Geometry check sheet. Reference: the model listing, model coordinates, mm. A direction names the side the tool comes from. Give positions to 0.01 mm unless a question says otherwise; leave off trailing zeros. Write each loop counter-clockwise with the first axis right and the second up, starting at its lowest first coordinate (ties: lowest second). Pieces come first, ordered by that corner, then holes.
(1) Mould release check, pull along X, two halves, no side actions. Record for faces 3 (the cylindrical face through (-1.923, 3.131, 107.933)), 4 (the flat face through (50.8, 3, -67)), 5 (the flat face through (-1, 6.35, -2)): +X half, -X half, draft (parallel to the pull), parting line (faces both ways), or undercut.
(2) Cross-section at A-A (x = 0). Record the boundary of the cut face in (y, z).
(3) Thickness scan on line 1 along Z through (x, y) = (-65.5, 3.5); line 2 along Z through (x, y) = (-7.5, 1); line 3 along X through (y, z) = (4.5, -36.83) (3 decimals). Record the ranges inside material, lowest first.
(4) Cross-section at D-D (y = 3). Count the separate pieces of the cut face and the enclosed holes in it, and give its area (3 significant figures).
(5) Depth check by flat-ended pin: P1, Ø1.5, axis at x = -40.5, y = 4.5, coming from the -Z side; P2, Ø3, axis at x = -45, y = 4, coming from the -Z side; P3, Ø3, axis at y = 4.5, z = -67, coming from the +X side. Enter the tip coordinate at first touch or a pass-through.
(6) Tool access check on faces 1 (the flat face through (-41, 3, -12.7)), 2 (the cylindrical face through (82.554, 3.131, 0.435)). Record the directions out of +Z, -Z, +X, -X, +Y, -Y that give a thin tool (end or side, any length) a straight path to the whole face; none if there is none.
(7) Cross-section at C-C (z = -21). Record the boundary of the cut face in (x, y), and give its area (3 significant figures).
(8) Cross-section at B-B (x = -28.5). Record the boundary of the cut face in (y, z), and give its area (3 significant figures).
```python
from build123d import *

# Parameters (mm, degrees)
SKETCH1_R           = 11.176
SKETCH1_R_2         = 3.175
SKETCH1_W           = 25.4
SKETCH1_H           = 6.35
SKETCH1_W_2         = 6.35
SKETCH1_H_2         = 25.4
SKETCH1_W_3         = 31.75
BOSS_EXTRUDE1_DEPTH = 6.35
SKETCH2_R           = 3.175
CUT_EXTRUDE1_DEPTH  = 6.35


with BuildPart() as part:
    # Sketch1 → Boss-Extrude1 (new body)
    with BuildSketch(Plane(origin=(0, 0, 0), x_dir=(1, 0, 0), z_dir=(0, 1, 0))):
        with BuildLine():
            ThreePointArc((-103.1875, -31.710287664), (0, -107.95), (103.1875, -31.710287664))
            ThreePointArc((103.1875, -31.710287664), (102.801250262, -27.013165433), (99.284117647, -23.8759813))
            ThreePointArc((99.284117647, -23.8759813), (82.55, 0), (99.284117647, 23.8759813))
            ThreePointArc((99.284117647, 23.8759813), (102.801250262, 27.013165433), (103.1875, 31.710287664))
            ThreePointArc((103.1875, 31.710287664), (0, 107.95), (-103.1875, 31.710287664))
            ThreePointArc((-103.1875, 31.710287664), (-102.801250262, 27.013165433), (-99.284117647, 23.8759813))
            ThreePointArc((-99.284117647, 23.8759813), (-82.55, 0), (-99.284117647, -23.8759813))
            ThreePointArc((-99.284117647, -23.8759813), (-102.801250262, -27.013165433), (-103.1875, -31.710287664))
        make_face()
        with Locations((0, 51.308)):
            Circle(SKETCH1_R, mode=Mode.SUBTRACT)
        with Locations((13.97, 36.83)):
            Circle(SKETCH1_R_2, mode=Mode.SUBTRACT)
        with Locations((-13.97, 36.83)):
            Circle(SKETCH1_R_2, mode=Mode.SUBTRACT)
        with Locations((-38.1, 66.675)):
            Rectangle(SKETCH1_W, SKETCH1_H, mode=Mode.SUBTRACT)
        with Locations((38.1, 66.675)):
            Rectangle(SKETCH1_W, SKETCH1_H, mode=Mode.SUBTRACT)
        with Locations((-38.1, -66.675)):
            Rectangle(SKETCH1_W, SKETCH1_H, mode=Mode.SUBTRACT)
        with Locations((38.1, -66.675)):
            Rectangle(SKETCH1_W, SKETCH1_H, mode=Mode.SUBTRACT)
        with Locations((41.275, -25.4)):
            Rectangle(SKETCH1_W_2, SKETCH1_H_2, mode=Mode.SUBTRACT)
        with Locations((41.275, 25.4)):
            Rectangle(SKETCH1_W_2, SKETCH1_H_2, mode=Mode.SUBTRACT)
        with Locations((-41.275, -25.4)):
            Rectangle(SKETCH1_W_2, SKETCH1_H_2, mode=Mode.SUBTRACT)
        with Locations((-41.275, 25.4)):
            Rectangle(SKETCH1_W_2, SKETCH1_H_2, mode=Mode.SUBTRACT)
        with Locations((0, 73.025)):
            Rectangle(SKETCH1_W_3, SKETCH1_H, mode=Mode.SUBTRACT)
        with Locations((0, -73.025)):
            Rectangle(SKETCH1_W_3, SKETCH1_H, mode=Mode.SUBTRACT)
    extrude(amount=BOSS_EXTRUDE1_DEPTH)

    # Sketch2 → Cut-Extrude1 (cut)
    with BuildSketch(Plane.XZ):
        with Locations((-66.8782, 66.8782)):
            Circle(SKETCH2_R)
        with Locations((66.8782, 66.8782)):
            Circle(SKETCH2_R)
        with Locations((66.8782, -66.8782)):
            Circle(SKETCH2_R)
        with Locations((-66.8782, -66.8782)):
            Circle(SKETCH2_R)
    extrude(amount=-CUT_EXTRUDE1_DEPTH, mode=Mode.SUBTRACT)


solid = part.part
```
Reply:
1. face 3: parting line
1. face 4: undercut
1. face 5: draft
2. outline: (0, -107.95) - (6.35, -107.95) - (6.35, -76.2) - (0, -76.2) - close; (0, -69.85) - (6.35, -69.85) - (6.35, -62.48) - (0, -62.48) - close; (0, -40.13) - (6.35, -40.13) - (6.35, 69.85) - (0, 69.85) - close; (0, 76.2) - (6.35, 76.2) - (6.35, 107.95) - (0, 107.95) - close
3. line 1: z = -85.81 to -69.74, -64.02 to 64.02, 69.74 to 85.81
3. line 2: z = -107.69 to -76.2, -69.85 to -59.59, -43.02 to 69.85, 76.2 to 107.69
3. line 3: x = -101.473 to -44.45, -38.1 to -17.145, -10.795 to 10.795, 17.145 to 38.1, 44.45 to 101.473
4. separate pieces: 1
4. enclosed holes: 17
4. area: 32,400 mm2
5. P1: stops at z = -100.37
5. P2: stops at z = -98.8
5. P3: stops at x = 85.81
6. face 1: +Y, -Y
6. face 2: +X, +Y, -Y
7. outline: (-93.66, 0) - (-44.45, 0) - (-44.45, 6.35) - (-93.66, 6.35) - close; (-38.1, 0) - (38.1, 0) - (38.1, 6.35) - (-38.1, 6.35) - close; (44.45, 0) - (93.66, 0) - (93.66, 6.35) - (44.45, 6.35) - close
7. area: 1,110 mm2
8. outline: (0, -104.12) - (6.35, -104.12) - (6.35, -69.85) - (0, -69.85) - close; (0, -63.5) - (6.35, -63.5) - (6.35, 63.5) - (0, 63.5) - close; (0, 69.85) - (6.35, 69.85) - (6.35, 104.12) - (0, 104.12) - close
8. area: 1,240 mm2
